from build123d import *

# Parameters (mm, degrees)
F0_R      = 9.525
F1_DEPTH  = 6.35
F2_R      = 9.525
F3_DEPTH  = 6.35
F5_DEPTH  = 9.525
F6_R      = 9.525
F7_DEPTH  = 11.176
F9_DEPTH  = 8.001
F10_R     = 1.7272
F11_DEPTH = 31.75
F13_DEPTH = 3.175
F14_DEPTH = 3.175
F19_R     = 1.7272
F20_DEPTH = 25.4
F21_R     = 1.7272
F22_DEPTH = 25.4
F26_DEPTH = 25.4
F28_DEPTH = 25.4


with BuildPart() as f1:
    # F0 (on Top) → F1 (new body)
    with BuildSketch(Plane.XY):
        with BuildLine():
            ThreePointArc((-9.514346, 0), (-14.164026, -11.22532), (-25.389346, -15.875))
            Line((-25.389346, -15.875), (28.585654, -15.875))
            Line((28.585654, -15.875), (28.585654, 15.875))
            Line((28.585654, 15.875), (-25.389346, 15.875))
            ThreePointArc((-25.389346, 15.875), (-14.164026, 11.22532), (-9.514346, 0))
        make_face()
        with BuildLine():
            ThreePointArc((-25.389346, 15.875), (-41.264346, 0), (-25.389346, -15.875))
            ThreePointArc((-25.389346, -15.875), (-14.164026, -11.22532), (-9.514346, 0))
            ThreePointArc((-9.514346, 0), (-14.164026, 11.22532), (-25.389346, 15.875))
        make_face()
        with Locations((-25.389346, 0)):
            Circle(F0_R, mode=Mode.SUBTRACT)
    extrude(amount=F1_DEPTH)

    # F2 (on face) → F3 (join)
    with BuildSketch(Plane.XY.offset(6.35)):
        with BuildLine():
            ThreePointArc((-25.389346, -15.875), (-14.164026, -11.22532), (-9.514346, 0))
            ThreePointArc((-9.514346, 0), (-14.164026, 11.22532), (-25.389346, 15.875))
            ThreePointArc((-25.389346, 15.875), (-41.264346, 0), (-25.389346, -15.875))
        make_face()
        with Locations((-25.389346, 0)):
            Circle(F2_R, mode=Mode.SUBTRACT)
    extrude(amount=F3_DEPTH)

    # F4 (on face) → F5 (join)
    with BuildSketch(Plane.YZ.offset(28.585654)):
        with BuildLine():
            Line((-15.875, 25.4), (-15.875, 0))
            Line((-15.875, 0), (15.875, 0))
            Line((15.875, 0), (15.875, 25.4))
            ThreePointArc((15.875, 25.4), (0, 41.275), (-15.875, 25.4))
        make_face()
    extrude(amount=-F5_DEPTH)

    # F6 (on face) → F7 (join)
    with BuildSketch(Plane.YZ.offset(28.585654)):
        with Locations((0, 25.4)):
            Circle(F6_R)
    extrude(amount=F7_DEPTH)

    # F8 (on face) → F9 (cut)
    with BuildSketch(Plane.YZ.offset(28.585654)):
        with BuildLine():
            Line((-10.3505, 6.35), (10.3505, 6.35))
            ThreePointArc((10.3505, 6.35), (10.889315, 6.573185), (11.1125, 7.112))
            Line((11.1125, 7.112), (11.1125, 13.462))
            ThreePointArc((11.1125, 13.462), (10.889315, 14.000815), (10.3505, 14.224))
            Line((10.3505, 14.224), (-10.3505, 14.224))
            ThreePointArc((-10.3505, 14.224), (-10.889315, 14.000815), (-11.1125, 13.462))
            Line((-11.1125, 13.462), (-11.1125, 7.112))
            ThreePointArc((-11.1125, 7.112), (-10.889315, 6.573185), (-10.3505, 6.35))
        make_face()
    extrude(amount=-F9_DEPTH, mode=Mode.SUBTRACT)

    # F10 (on face) → F11 (cut)
    with BuildSketch(Plane.XZ.offset(15.875)):
        with Locations((25.410654, 10.287)):
            Circle(F10_R)
    extrude(amount=-F11_DEPTH, mode=Mode.SUBTRACT)

    # F19 (on face) → F20 (cut)
    with BuildSketch(Plane(origin=(-12.694673, 12.694673, 0), x_dir=(0.707107, 0.707107, 0), z_dir=(0.707107, -0.707107, 0))):
        with Locations((-17.916348, 6.420591)):
            Circle(F19_R)
    extrude(amount=-F20_DEPTH, mode=Mode.SUBTRACT)

    # F21 (on face) → F22 (cut)
    with BuildSketch(Plane(origin=(-12.694673, -12.694673, 0), x_dir=(-0.707107, 0.707107, 0), z_dir=(0.707107, 0.707107, 0))):
        with Locations((17.901907, 6.418147)):
            Circle(F21_R)
    extrude(amount=-F22_DEPTH, mode=Mode.SUBTRACT)

    # F25 (on face) → F26 (join)
    with BuildSketch(Plane.XY.offset(6.35)):
        with BuildLine():
            ThreePointArc((-9.835086, 3.175), (-9.514346, 0), (-9.835086, -3.175))
            Line((-9.835086, -3.175), (19.060654, -3.175))
            Line((19.060654, -3.175), (19.060654, 3.175))
            Line((19.060654, 3.175), (-9.835086, 3.175))
        make_face()
    extrude(amount=F26_DEPTH)

    # F27 (on face) → F28 (cut)
    with BuildSketch(Plane.XZ.offset(3.175)):
        with BuildLine():
            Line((-6.43225, 11.53927), (19.060654, 25.4))
            Line((19.060654, 25.4), (19.060654, 31.75))
            Line((19.060654, 31.75), (-9.835086, 31.75))
            Line((-9.835086, 31.75), (-9.835086, 12.7))
            ThreePointArc((-9.835086, 12.7), (-8.423755, 11.269205), (-6.43225, 11.53927))
        make_face()
    extrude(amount=-F28_DEPTH, mode=Mode.SUBTRACT)


with BuildPart() as f13:
    # F12 (on Front) → F13 (new body, symmetric)
    with BuildSketch(Plane.XZ):
        with BuildLine():
            Line((18.935824, 6.271193), (19.060654, 25.4))
            Line((19.060654, 25.4), (-5.57432, 8.746564))
            ThreePointArc((-5.57432, 8.746564), (-8.13987, 8.590052), (-9.515413, 10.761324))
            Line((-9.515413, 10.761324), (-9.515413, 6.271193))
            Line((-9.515413, 6.271193), (18.935824, 6.271193))
        make_face()
    extrude(amount=F13_DEPTH, both=True)


with BuildPart() as f14:
    # F12 (on Front) → F14 (new body, symmetric)
    with BuildSketch(Plane.XZ):
        with BuildLine():
            Line((18.935824, 6.271193), (19.060654, 25.4))
            Line((19.060654, 25.4), (-5.57432, 8.746564))
            ThreePointArc((-5.57432, 8.746564), (-8.13987, 8.590052), (-9.515413, 10.761324))
            Line((-9.515413, 10.761324), (-9.515413, 6.271193))
            Line((-9.515413, 6.271193), (18.935824, 6.271193))
        make_face()
    extrude(amount=F14_DEPTH, both=True)


solid = f1.part
Source: CAD feature listing. Evaluate the final solid. Frame: model axes, mm. A direction names the side the tool comes from. Coordinates: 2 decimals unless noted, no trailing zeros. Order: outer loops, then holes, each group sorted by start corner. A loop starts at its lowest first (then second) coordinate and runs counter-clockwise, first axis right, second up.
Item 1: Pull-direction query (Y, two-part tool) for faces 1 (the face through (-34.898, -8.268, 7.875)), 2 (the face through (28.586, 3, 16)), 3 (the face through (25, 0, 6.35)), 4 (the face through (8, 3.175, 14)); classes: pulls with the +Y half, pulls with the -Y half, needs draft (parallel to the pull), parting line crosses it, or undercut.
Output values:
face 1: undercut
face 2: needs draft
face 3: undercut
face 4: pulls with the +Y half
Item 2: Cut plane A-A (y = 0). Return loops of the section in (x, z) (3 decimals), plus the area to 3 significant figures.
Output values:
outline: (-41.264, 0) - (-34.914, 0) - (-34.914, 12.7) - (-41.264, 12.7) - close; (-15.864, 0) - (28.586, 0) - (28.586, 6.35) - (20.585, 6.35) - (20.585, 14.224) - (28.586, 14.224) - (28.586, 15.875) - (39.762, 15.875) - (39.762, 34.925) - (28.586, 34.925) - (28.586, 41.275) - (19.061, 41.275) - (19.061, 25.4) - (-6.432, 11.539) arc R2.248 cw to (-9.835, 12.7) - (-15.864, 12.7) - close
area: 1,210 mm2
Item 3: Material intervals for line 1 (X direction, y = -6.5, z = 12); line 2 (Y direction, x = 2, z = 7) (3 decimals); line 3 (Z direction, x = -16.5, y = -11.5), sorted ascending.
Output values:
line 1: x = -39.87 to -32.35, -18.43 to -10.91, 19.06 to 20.58
line 2: y = -3.175 to 3.175
line 3: z = 0 to 12.7
Item 4: Set-up query: faces 5 (the face through (-18.8, 7.3, 12.7)), 6 (the face through (34.1, -2.06, 16.1)), 7 (the face through (19.061, -4, 24)), 8 (the face through (1, -9, 6.35)), 9 (the face through (-16.59, -3.65, 6.26)). Return all of +Z, -Z, +X, -X, +Y, -Y with unobstructed straight access to the full face (end or side cutting, diameter ignored); none if empty.
Output values:
face 5: +Z, -X, +Y, -Y
face 6: +X
face 7: +Z
face 8: +Z, -Y
face 9: +Z, -Z
Item 5: First-contact query: P1, Ø12, axis at y = 11, z = 12.5, coming from the +X side; P2, Ø6, axis at x = -9, z = 12.5, coming from the +Y side; P3, Ø6.5, axis at x = -8, y = -12.5, coming from the +Z side. Flat tips, straight axial feed; report the tip coordinate or a pass-through.
Output values:
P1: stops at x = 28.59
P2: stops at y = 8.53
P3: stops at z = 6.35
Item 6: Cut plane D-D (y = 4). Return loops of the section in (x, z).
Output values:
outline: (-40.75, 0) - (-34.03, 0) - (-34.03, 12.7) - (-40.75, 12.7) - close; (-16.74, 0) - (28.59, 0) - (28.59, 6.35) - (20.58, 6.35) - (20.58, 14.22) - (28.59, 14.22) - (28.59, 16.76) - (39.76, 16.76) - (39.76, 34.04) - (28.59, 34.04) - (28.59, 40.76) - (19.06, 40.76) - (19.06, 6.35) - (-10.03, 6.35) - (-10.03, 12.7) - (-16.74, 12.7) - close
Item 7: Cut plane C-C (x = -20). Return loops of the section in (y, z) (3 decimals), plus the area to 3 significant figures.
Output values:
outline: (-15.875, 0) - (-7.854, 0) - (-7.854, 12.7) - (-14.932, 12.7) - (-14.932, 6.35) - (-15.875, 6.35) - close; (7.854, 0) - (15.875, 0) - (15.875, 6.35) - (14.932, 6.35) - (14.932, 12.7) - (7.854, 12.7) - close
area: 192 mm2
